from build123d import *

# Parameters (mm, degrees)
PAD003_DEPTH    = 8
SKETCH007_R     = 14.75
PAD004_DEPTH    = 18.5
PAD005_DEPTH    = 10
SKETCH009_R     = 2.8
POCKET002_DEPTH = 36.501
CHAMFER_SIZE    = 1


with BuildPart() as part:
    # Sketch006 → Pad003 (new body)
    with BuildSketch(Plane.XY):
        Polygon((0, -11.25833), (9.75, -5.629165), (9.75, 5.629165), (0, 11.25833), (-9.75, 5.629165), (-9.75, -5.629165), align=None)
    extrude(amount=PAD003_DEPTH)

    # Sketch007 (on Face8 of Pad003) → Pad004 (join)
    with BuildSketch(Plane.XY.offset(8)):
        Circle(SKETCH007_R)
    extrude(amount=PAD004_DEPTH)

    # Sketch008 (on Face3 of Pad004) → Pad005 (join)
    with BuildSketch(Plane.XY.offset(26.5)):
        with BuildLine():
            ThreePointArc((7.111111, 18.693103), (-20, 0), (7.111111, -18.693103))
            Line((46.422222, -3.738621), (7.111111, -18.693103))
            ThreePointArc((46.422222, -3.738621), (49, 0), (46.422222, 3.738621))
            Line((46.422222, 3.738621), (7.111111, 18.693103))
        make_face()
    extrude(amount=PAD005_DEPTH)

    # Sketch009 (on Face5 of Pad005) → Pocket002 (cut, through all)
    with BuildSketch(Plane.XY.offset(36.5)):
        Circle(SKETCH009_R)
    extrude(amount=-POCKET002_DEPTH, mode=Mode.SUBTRACT)

    # Chamfer
    chamfer_edges = [part.edges().sort_by_distance(p)[0] for p in [
        (49, 0, 36.5),
        (26.766667, -11.215862, 36.5),
        (26.766667, 11.215862, 36.5),
        (-20, 0, 36.5),
        (-2.8, 0, 36.5),
        (26.766667, -11.215862, 26.5),
        (4.875, -8.443748, 0),
        (-4.875, -8.443748, 0),
        (9.75, 0, 0),
        (-9.75, 0, 0),
        (4.875, 8.443748, 0),
        (-4.875, 8.443748, 0),
        (-2.8, 0, 0),
    ]]
    chamfer(chamfer_edges, length=CHAMFER_SIZE)


solid = part.part
Work out the finished part from the listing and answer in its coordinate system (mm). A direction names the side the tool comes from. Give positions to 0.01 mm unless a question says otherwise; leave off trailing zeros. Loops run counter-clockwise (first coordinate to the right, second up) from the corner with the lowest first, then second, coordinate; pieces in that order, holes last. Notation, with made-up numbers: (89.5, -26.5) -> (125.5, -26.5) arc R28 ccw to (125.5, 7.5) -> close; hole circle Ø3 at (70.25, 57). An arc over 180 degrees is marked (long way). Use a Markdown table: item, result. Add a question column.
1. Section B-B on z = 30.5 is taken. Determine the outline of the cut face in (x, y).
2. Flat-ended cylindrical pins translate along their axes: pin 1 Ø1 at (x, y) = (33.5, -1.5) entering from -Z; pin 2 Ø4 at (x, z) = (25.5, 30.5) entering from -Y; pin 3 Ø5 at (y, z) = (-9, 32) entering from -X; pin 4 Ø5 at (x, y) = (0, 0) entering from +Z. Find the tip coordinate at first contact, or state that the pin passes through.
3. Determine the mould class of faces 5 (the flat face through (9.75, 0, 4)), 6 (the flat face through (-4.943, -8.404, 4.451)), 7 (the cylindrical face through (14.07, 4.43, 17.12)) for opening direction X: released by +X, released by -X, zero draft, split by the parting line, or undercut.
4. Find the intervals of material crossed by probe 1 along Y at (x, z) = (0, 20); probe 2 along Z at (x, y) = (32.5, -1); probe 3 along Z at (x, y) = (-8.5, -11.5), in increasing order.
5. Section C-C on x = 31.5 is taken. Determine the outline of the cut face in (y, z).
6. Section D-D on z = 23.5 is taken. Determine the outline of the cut face in (x, y), and give its area (3 significant figures).
7. Section A-A on y = 0 is taken. Determine the outline of the cut face in (x, z).
8. For faces 1 (the flat face through (4.81, -8.48, 4.45)), 2 (the flat face through (4.943, 8.404, 4.451)), 3 (the flat face through (-9.75, 0, 4)), 4 (the flat face through (-3, -10, 8)), determine the directions among +Z, -Z, +X, -X, +Y, -Y from which every point of the face is accessible in a straight line to the end or side of a thin tool.
Results below:
| question | item | result |
|---|---|---|
| 1 | outline | (7.11, -18.69) -> (46.42, -3.74) arc R4 ccw to (46.42, 3.74) -> (7.11, 18.69) arc R20 ccw (long way) to start; hole circle Ø5.6 at (0, 0) |
| 2 | pin 1 | stops at z = 26.5 |
| 2 | pin 2 | stops at y = -12.46 |
| 2 | pin 3 | stops at x = -18.91 |
| 2 | pin 4 | passes through |
| 3 | face 5 | released by +X |
| 3 | face 6 | released by -X |
| 3 | face 7 | split by the parting line |
| 4 | probe 1 | y = -14.75 to -2.8, 2.8 to 14.75 |
| 4 | probe 2 | z = 26.5 to 36.5 |
| 4 | probe 3 | z = 8 to 36.5 |
| 5 | outline | (-9.42, 27.5) -> (-8.35, 26.5) -> (8.35, 26.5) -> (9.42, 27.5) -> (9.42, 35.5) -> (8.35, 36.5) -> (-8.35, 36.5) -> (-9.42, 35.5) -> close |
| 6 | outline | circle Ø29.5 at (0, 0); hole circle Ø5.6 at (0, 0) |
| 6 | area | 659 mm^2 |
| 7 | outline | (-20, 27.5) -> (-19, 26.5) -> (-14.75, 26.5) -> (-14.75, 8) -> (-9.75, 8) -> (-9.75, 1) -> (-8.75, 0) -> (-3.8, 0) -> (-2.8, 1) -> (-2.8, 35.5) -> (-3.8, 36.5) -> (-19, 36.5) -> (-20, 35.5) -> close; (2.8, 1) -> (3.8, 0) -> (8.75, 0) -> (9.75, 1) -> (9.75, 8) -> (14.75, 8) -> (14.75, 26.5) -> (48, 26.5) -> (49, 27.5) -> (49, 35.5) -> (48, 36.5) -> (3.8, 36.5) -> (2.8, 35.5) -> close |
| 8 | face 1 | -Z, +X, -Y |
| 8 | face 2 | -Z, +X, +Y |
| 8 | face 3 | -Z, -X, +Y, -Y |
| 8 | face 4 | -Z |
